The model under review builds one solid part; all positions refer to its coordinate system, in mm. Face numbers are marked on the shaded views. A direction names the side the tool comes from. Give positions to 0.01 mm unless a question says otherwise; leave off trailing zeros. Order: outer loops, then holes, each group sorted by start corner. A loop starts at its lowest first (then second) coordinate and runs counter-clockwise, first axis right, second up. Notation, with made-up numbers: (37, -31) -> (73, -31) arc R9 cw to (73, -16) -> close; hole circle Ø8 at (5, -38.75). An arc over 180 degrees is marked (long way). Answer as a JSON object with one key per item and string values. Group by question number.
from build123d import *

# Parameters (mm, degrees)
SKETCH1_R                                           = 14
BOSS_EXTRUDE1_DEPTH                                 = 24
SKETCH2_R                                           = 23
SKETCH2_R_2                                         = 9
BOSS_EXTRUDE2_DEPTH                                 = 8
SKETCH3_R                                           = 9
CUT_EXTRUDE1_DEPTH                                  = 41.422765863
CBORE_FOR_M4_HEX_SOCKET_HEAD_CAP_SCREW1_D           = 4.5
CBORE_FOR_M4_HEX_SOCKET_HEAD_CAP_SCREW1_CBORE_D     = 8
CBORE_FOR_M4_HEX_SOCKET_HEAD_CAP_SCREW1_CBORE_DEPTH = 4.4
CIRPATTERN1_COUNT                                   = 3
FILLET1_R                                           = 2
FILLET2_R                                           = 1


with BuildPart() as part:
    # Sketch1 → Boss-Extrude1 (new body)
    with BuildSketch(Plane.XY):
        Circle(SKETCH1_R)
    extrude(amount=BOSS_EXTRUDE1_DEPTH)

    # Sketch2 → Boss-Extrude2 (add)
    with BuildSketch(Plane.XY.offset(24)):
        Circle(SKETCH2_R)
        Circle(SKETCH2_R_2, mode=Mode.SUBTRACT)
    extrude(amount=BOSS_EXTRUDE2_DEPTH)

    # Sketch3 → Cut-Extrude1 (cut, through all)
    with BuildSketch(Plane.XY.offset(24)):
        Circle(SKETCH3_R)
    extrude(amount=-CUT_EXTRUDE1_DEPTH, mode=Mode.SUBTRACT)

    # CBORE for M4 Hex Socket Head Cap Screw1 (through all)
    with Locations(Plane.XY.offset(32)):
        with Locations((0, -18)):
            cbore_for_m4_hex_socket_head_cap_screw1 = CounterBoreHole(CBORE_FOR_M4_HEX_SOCKET_HEAD_CAP_SCREW1_D / 2, CBORE_FOR_M4_HEX_SOCKET_HEAD_CAP_SCREW1_CBORE_D / 2, CBORE_FOR_M4_HEX_SOCKET_HEAD_CAP_SCREW1_CBORE_DEPTH)

    # CirPattern1: CBORE for M4 Hex Socket Head Cap Screw1 ×3 about axis
    cirpattern1_axis = Axis((0, 0, 0), (0, 0, 1))
    for i in range(1, CIRPATTERN1_COUNT):
        add(cbore_for_m4_hex_socket_head_cap_screw1.rotate(cirpattern1_axis, i * 360 / CIRPATTERN1_COUNT), mode=Mode.SUBTRACT)

    # Fillet1
    fillet1_edges = [part.edges().sort_by_distance(p)[0] for p in [
        (-9, 0, 32),
    ]]
    fillet(fillet1_edges, radius=FILLET1_R)

    # Fillet2
    fillet2_edges = [part.edges().sort_by_distance(p)[0] for p in [
        (-14, 0, 24),
    ]]
    fillet(fillet2_edges, radius=FILLET2_R)


solid = part.part
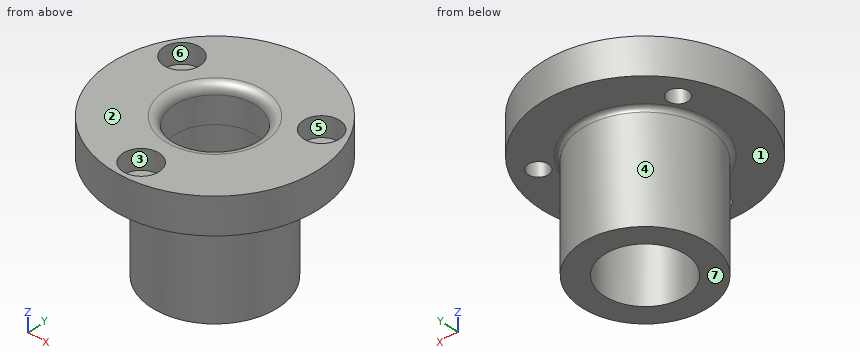
1. For probe 1 along Y at (x, z) = (0, 29); probe 2 along Y at (x, z) = (0, 2); probe 3 along Y at (x, z) = (1, 7), list the stretches that pass through material, from the lowest coordinate up. Write a range as [from, to].
2. Machinability: for the marked faces 1, 2 and 3, which of the approach directions +Z, -Z, +X, -X, +Y, -Y give a long, thin tool a straight path to every point of the face, cutting with its end or side? Answer none if there is none.
3. For pin 1 (4 mm diameter, centred on x = -15.5, y = 8, fed in from +Z); pin 2 (16 mm diameter, centred on x = 0, y = 0, fed in from -Z); pin 3 (1.5 mm diameter, centred on y = -11, z = 4, fed in from -X); pin 4 (4 mm diameter, centred on y = 4, z = 18, fed in from -X), all flat-tipped, find the tip position at first contact; note any pin that passes through.
4. Take a section at A-A on x = 0. Give the boundary of the cut face in (y, z), plus the area to 3 significant figures.
5. Take a section at C-C on z = 13. Give the boundary of the cut face in (x, y), plus the area to 3 significant figures.
6. Take a section at B-B on y = 0. Give the boundary of the cut face in (x, z), plus the area to 3 significant figures.
7. Take a section at D-D on y = -18. Give the boundary of the cut face in (x, z), plus the area to 3 significant figures.
8. Draft analysis for pull direction X (two halves, no side actions). For the marked faces 4, 5, 6 and 7, state which applies: pulls with the +X half, pulls with the -X half, needs draft (parallel to the pull), parting line crosses it, or undercut.
Checks:
{
 "1": {"probe 1": "y = [-23, -22], [-14, -9], [9, 23]", "probe 2": "y = [-14, -9], [9, 14]", "probe 3": "y = [-13.96, -8.94], [8.94, 13.96]"},
 "2": {"face 1": "-Z", "face 2": "+Z, +X, -X, +Y, -Y", "face 3": "+Z"},
 "3": {"pin 1": "stops at z = 27.6", "pin 2": "passes through", "pin 3": "stops at x = -9.54", "pin 4": "stops at x = -13.86"},
 "4": {"outline": "(-23, 24) -> (-20.25, 24) -> (-20.25, 27.6) -> (-22, 27.6) -> (-22, 32) -> (-23, 32) -> close; (-15.75, 24) -> (-15, 24) arc R1 cw to (-14, 23) -> (-14, 0) -> (-9, 0) -> (-9, 30) arc R2 ccw to (-11, 32) -> (-14, 32) -> (-14, 27.6) -> (-15.75, 27.6) -> close; (9, 0) -> (14, 0) -> (14, 23) arc R1 cw to (15, 24) -> (23, 24) -> (23, 32) -> (11, 32) arc R2 ccw to (9, 30) -> close", "area": "411 mm2"},
 "5": {"outline": "circle Ø28 at (0, 0); hole circle Ø18 at (0, 0)", "area": "361 mm2"},
 "6": {"outline": "(-23, 24) -> (-15, 24) arc R1 cw to (-14, 23) -> (-14, 0) -> (-9, 0) -> (-9, 30) arc R2 ccw to (-11, 32) -> (-23, 32) -> close; (9, 0) -> (14, 0) -> (14, 23) arc R1 cw to (15, 24) -> (23, 24) -> (23, 32) -> (11, 32) arc R2 ccw to (9, 30) -> close", "area": "463 mm2"},
 "7": {"outline": "(-14.32, 24) -> (-2.25, 24) -> (-2.25, 27.6) -> (-4, 27.6) -> (-4, 32) -> (-14.32, 32) -> close; (2.25, 24) -> (14.32, 24) -> (14.32, 32) -> (4, 32) -> (4, 27.6) -> (2.25, 27.6) -> close", "area": "178 mm2"},
 "8": {"face 4": "parting line crosses it", "face 5": "undercut", "face 6": "undercut", "face 7": "needs draft"}
}
